Geometry: see drawing. Coordinates: mm, zero at the bounding-box minimum. Round coordinates to 2 decimals unless told otherwise and drop trailing zeros. Loops run counter-clockwise (first coordinate to the right, second up) from the corner with the lowest first, then second, coordinate; pieces in that order, holes last. Notation, with made-up numbers: M 77,14 L 130,14 A29 ccw 130,45 Z; hole C -15,-34.75 d6. An arc over 180 degrees is marked long. Answer as a JSON object with one key per item and string values.
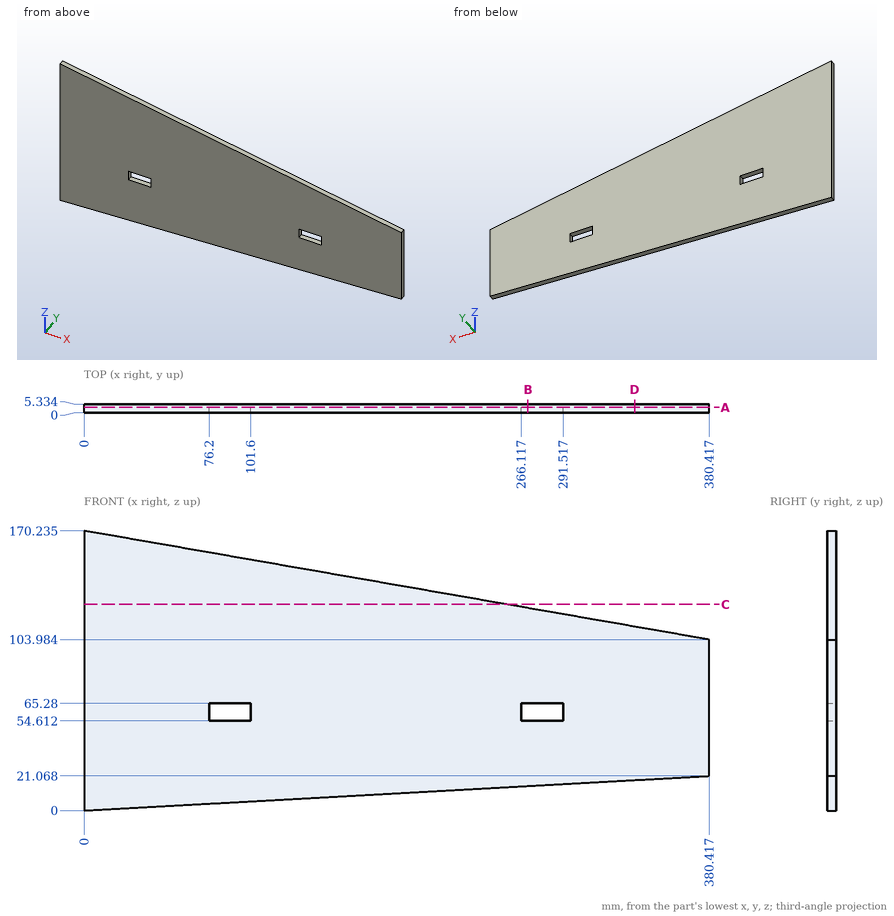
1) Section query A-A (y = 3.35). Return the cut outline in (x, z) (1 decimal), and give its area (3 significant figures).
Results:
{"outline": "M 0,0 L 380.4,21.1 L 380.4,104 L 0,170.2 Z; hole M 76.2,54.6 L 101.6,54.6 L 101.6,65.3 L 76.2,65.3 Z; hole M 266.1,54.6 L 291.5,54.6 L 291.5,65.3 L 266.1,65.3 Z", "area": "47,600 mm2"}
2) Ray query, line 1 (X direction, y = 3.7, z = 55); line 2 (Z direction, x = 97, y = 0.2); line 3 (Z direction, x = 284, y = 3.6) (1 decimal). Return the intervals inside material, ascending.
Results:
{"line 1": "0 to 76.2, 101.6 to 266.12, 291.52 to 380.42", "line 2": "5.37 to 54.61, 65.28 to 153.34", "line 3": "15.7 to 54.6, 65.3 to 120.8"}
3) Pin query (flat end, axial travel): P1, Ø1.6, axis at x = 284, y = 3, coming from the -Z side; P2, Ø2.5, axis at x = 279.5, y = 3.5, coming from the +Z side; P3, Ø1.5, axis at x = 164, y = 4, coming from the +Z side (1 decimal). Return the tip coordinate at first contact, or that it passes through.
Results:
{"P1": "z = 15.68", "P2": "z = 121.78", "P3": "z = 141.8"}
4) Section query B-B (x = 270). Return the cut outline in (y, z).
Results:
{"outline": "M 0,14.95 L 5.33,14.95 L 5.33,54.61 L 0,54.61 Z; M 0,65.28 L 5.33,65.28 L 5.33,123.21 L 0,123.21 Z"}
5) Section query D-D (x = 335). Return the cut outline in (y, z).
Results:
{"outline": "M 0,18.55 L 5.33,18.55 L 5.33,111.89 L 0,111.89 Z"}
6) Section query C-C (z = 125.5). Return the cut outline in (x, y), and give its area (3 significant figures).
Results:
{"outline": "M 0,0 L 256.87,0 L 256.87,5.33 L 0,5.33 Z", "area": "1,370 mm2"}
